from build123d import *

# Parameters (mm, degrees)
SKETCH1_W           = 136
SKETCH1_H           = 12
SKETCH1_R           = 2.1
SKETCH1_R_2         = 5
SKETCH1_R_3         = 2.7
BOSS_EXTRUDE1_DEPTH = 5
SKETCH2_W           = 96
SKETCH2_H           = 3
CUT_EXTRUDE1_DEPTH  = 12
SKETCH1_3_R         = 5
CUT_EXTRUDE2_DEPTH  = 3


with BuildPart() as part:
    # Sketch1 → Boss-Extrude1 (new body)
    with BuildSketch(Plane.XY):
        Rectangle(SKETCH1_W, SKETCH1_H)
        with Locations((25, 0)):
            Circle(SKETCH1_R, mode=Mode.SUBTRACT)
        with Locations((-58, 0)):
            Circle(SKETCH1_R_2, mode=Mode.SUBTRACT)
        with Locations((-25, 0)):
            Circle(SKETCH1_R, mode=Mode.SUBTRACT)
        with Locations((58, 0)):
            Circle(SKETCH1_R_2, mode=Mode.SUBTRACT)
        with Locations((-58, 0)):
            Circle(SKETCH1_R_2)
        with Locations((-58, 0)):
            Circle(SKETCH1_R_3, mode=Mode.SUBTRACT)
        with Locations((58, 0)):
            Circle(SKETCH1_R_2)
        with Locations((58, 0)):
            Circle(SKETCH1_R_3, mode=Mode.SUBTRACT)
    extrude(amount=BOSS_EXTRUDE1_DEPTH)

    # Sketch2 → Cut-Extrude1 (cut)
    with BuildSketch(Plane.XZ.offset(6)):
        with Locations((0, 3.5)):
            Rectangle(SKETCH2_W, SKETCH2_H)
    extrude(amount=-CUT_EXTRUDE1_DEPTH, mode=Mode.SUBTRACT)

    # Sketch1<3> → Cut-Extrude2 (cut)
    with BuildSketch(Plane.XY):
        with Locations((-58, 0)):
            Circle(SKETCH1_3_R)
        with Locations((58, 0)):
            Circle(SKETCH1_3_R)
    extrude(amount=CUT_EXTRUDE2_DEPTH, mode=Mode.SUBTRACT)


solid = part.part
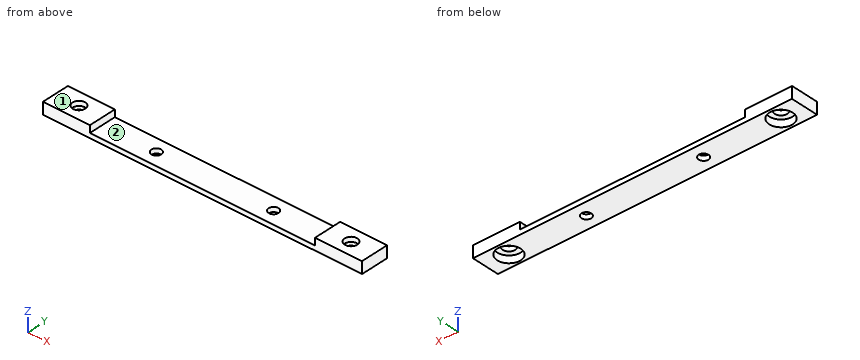
Geometry: final body of the model. Coordinates: model frame, mm. Face numbers are marked on the shaded views. Give positions to 0.01 mm unless a question says otherwise; leave off trailing zeros. Write each loop counter-clockwise with the first axis right and the second up, starting at its lowest first coordinate (ties: lowest second). Pieces come first, ordered by that corner, then holes. Notation, with made-up numbers: M -39,3.25 L 17,3.25 A31 cw 17,40.25 Z; hole C 84,68 d1. An arc over 180 degrees is marked long. Answer in a Markdown table with one row per item. Add a question column.
(1) Section C-C on z = 1.05. Return loops of the section in (x, y).
(2) Section D-D on x = 25. Return loops of the section in (y, z), and give its area (3 significant figures).
(3) First-contact query: pin 1 (6 mm diameter, centred on x = 58, y = 0, fed in from -Z); pin 2 (5.5 mm diameter, centred on x = -25, y = 0, fed in from +Z). Flat tips, straight axial feed; report the tip coordinate or a pass-through.
(4) Mould query, pull axis X, two halves, no side actions, for the marked faces 1 and 2. Classes: +X half, -X half, draft (parallel to the pull), parting line (faces both ways), or undercut.
(5) Section A-A on x = 58. Return loops of the section in (y, z), and give its area (3 significant figures).
(6) Ray query, line 1 (X direction, y = 0, z = 3.65); line 2 (X direction, y = 2.75, z = 0.95); line 3 (X direction, y = -2.25, z = 0.75). Return the intervals inside material, ascending.
(7) Section B-B on y = 0. State how many separate pieces and enclosed holes the cut face has, and give its area (3 significant figures).
Result set:
| question | item | result |
|---|---|---|
| 1 | outline | M -68,-6 L 68,-6 L 68,6 L -68,6 Z; hole C -58,0 d10; hole C -25,0 d4.2; hole C 25,0 d4.2; hole C 58,0 d10 |
| 2 | outline | M -6,0 L -2.1,0 L -2.1,2 L -6,2 Z; M 2.1,0 L 6,0 L 6,2 L 2.1,2 Z |
| 2 | area | 15.6 mm^2 |
| 3 | pin 1 | stops at z = 3 |
| 3 | pin 2 | stops at z = 2 |
| 4 | face 1 | draft |
| 4 | face 2 | undercut |
| 5 | outline | M -6,0 L -5,0 L -5,3 L -2.7,3 L -2.7,5 L -6,5 Z; M 2.7,3 L 5,3 L 5,0 L 6,0 L 6,5 L 2.7,5 Z |
| 5 | area | 19.2 mm^2 |
| 6 | line 1 | x = -68 to -60.7, -55.3 to -48, 48 to 55.3, 60.7 to 68 |
| 6 | line 2 | x = -68 to -62.18, -53.82 to 53.82, 62.18 to 68 |
| 6 | line 3 | x = -68 to -62.47, -53.53 to 53.53, 62.47 to 68 |
| 7 | separate pieces | 5 |
| 7 | enclosed holes | 0 |
| 7 | area | 294 mm^2 |
